from build123d import *
from build123d.topology import SkipClean

# Parameters (mm, degrees)
SKETCH1_W           = 95
SKETCH1_H           = 62
SKETCH1_R           = 1.7
BOSS_EXTRUDE1_DEPTH = 3
SKETCH2_W           = 75
SKETCH2_H           = 52
BOSS_EXTRUDE2_DEPTH = 28.85
SKETCH3_W           = 69
SKETCH3_H           = 25.85
CUT_EXTRUDE1_DEPTH  = 118.827935991
SKETCH4_W           = 69
SKETCH4_H           = 3
CUT_EXTRUDE2_DEPTH  = 118.827935991
SKETCH5_R           = 1.3
SKETCH5_W           = 32
SKETCH5_H           = 14
CUT_EXTRUDE3_DEPTH  = 118.827935991
SKETCH7_R           = 3
CUT_EXTRUDE5_DEPTH  = 118.827935991
SKETCH6_W           = 15
SKETCH6_H           = 9
SKETCH6_W_2         = 8
SKETCH6_H_2         = 10.5
CUT_EXTRUDE4_DEPTH  = 118.827935991
FILLET1_R           = 2
SKETCH8_R           = 2.5
SKETCH8_R_2         = 1.3
BOSS_EXTRUDE4_DEPTH = 4
FILLET2_R           = 5


with BuildPart() as part:
    # Sketch1 → Boss-Extrude1 (new body)
    with BuildSketch(Plane(origin=(0, 0, 0), x_dir=(1, 0, 0), z_dir=(0, 1, 0))):
        with Locations((47.5, 31)):
            Rectangle(SKETCH1_W, SKETCH1_H)
        with Locations(Location((90.04349796, 55.565, 0), (0, 0, 270))):
            Circle(SKETCH1_R, mode=Mode.SUBTRACT)
        with Locations(Location((90.04349796, 6.435, 0), (0, 0, 270))):
            Circle(SKETCH1_R, mode=Mode.SUBTRACT)
        with Locations(Location((4.95650204, 55.565, 0), (0, 0, 270))):
            Circle(SKETCH1_R, mode=Mode.SUBTRACT)
        with Locations(Location((4.95650204, 6.435, 0), (0, 0, 270))):
            Circle(SKETCH1_R, mode=Mode.SUBTRACT)
    extrude(amount=BOSS_EXTRUDE1_DEPTH)

    # Sketch2 → Boss-Extrude2 (add)
    with BuildSketch(Plane(origin=(0, 3, 0), x_dir=(1, 0, 0), z_dir=(0, 1, 0))):
        with Locations((47.5, 26)):
            Rectangle(SKETCH2_W, SKETCH2_H)
    extrude(amount=BOSS_EXTRUDE2_DEPTH)

    # Sketch3 → Cut-Extrude1 (cut, through all)
    with BuildSketch(Plane.XY):
        with Locations((47.5, 15.925)):
            Rectangle(SKETCH3_W, SKETCH3_H)
    extrude(amount=-CUT_EXTRUDE1_DEPTH, mode=Mode.SUBTRACT)

    # Sketch4 → Cut-Extrude2 (cut, through all)
    with BuildSketch(Plane.XY):
        with Locations((47.5, 1.5)):
            Rectangle(SKETCH4_W, SKETCH4_H)
    extrude(amount=-CUT_EXTRUDE2_DEPTH, mode=Mode.SUBTRACT)

    # Sketch5 → Cut-Extrude3 (cut, through all)
    with BuildSketch(Plane(origin=(0, 31.85, 0), x_dir=(1, 0, 0), z_dir=(0, 1, 0))):
        with Locations(Location((27.5, 46, 0), (0, 0, 270))):
            Circle(SKETCH5_R)
        with Locations(Location((27.5, 8, 0), (0, 0, 270))):
            Circle(SKETCH5_R)
        with Locations(Location((67.5, 8, 0), (0, 0, 270))):
            Circle(SKETCH5_R)
        with Locations(Location((67.5, 46, 0), (0, 0, 270))):
            Circle(SKETCH5_R)
        with Locations((47.5, 7)):
            Rectangle(SKETCH5_W, SKETCH5_H)
    extrude(amount=-CUT_EXTRUDE3_DEPTH, mode=Mode.SUBTRACT)

    # Sketch7 → Cut-Extrude5 (cut, through all)
    with BuildSketch(Plane(origin=(0, 31.85, 0), x_dir=(1, 0, 0), z_dir=(0, 1, 0))):
        with Locations((34, 10.8)):
            Circle(SKETCH7_R)
        with Locations((61, 10.8)):
            Circle(SKETCH7_R)
    extrude(amount=-CUT_EXTRUDE5_DEPTH, mode=Mode.SUBTRACT)

    # Sketch6 → Cut-Extrude4 (cut, through all)
    with BuildSketch(Plane(origin=(0, 31.85, 0), x_dir=(1, 0, 0), z_dir=(0, 1, 0))):
        with Locations((38.8, 47.5)):
            Rectangle(SKETCH6_W, SKETCH6_H)
        with Locations((68, 37.75)):
            Rectangle(SKETCH6_W_2, SKETCH6_H_2)
    extrude(amount=-CUT_EXTRUDE4_DEPTH, mode=Mode.SUBTRACT)

    # Fillet1
    fillet1_edges = [part.edges().sort_by_distance(p)[0] for p in [
        (10, 3, -26),
        (85, 3, -26),
        (10, 31.85, -26),
        (85, 31.85, -26),
        (13, 28.85, -26),
        (82, 28.85, -26),
        (13, 0, -31),
        (82, 0, -31),
    ]]
    fillet(fillet1_edges, radius=FILLET1_R)

    # Sketch8 → Boss-Extrude4 (add)
    # profile 1 of 4: a face of its own
    with SkipClean():  # the faces are left unmerged after this step: merging them gives an invalid solid
        with BuildSketch(Plane.XZ.offset(-28.85)):
            with Locations(Location((27.5, -8, 0), (0, 0, 90))):
                Circle(SKETCH8_R)
            with Locations(Location((27.5, -8, 0), (0, 0, 90))):
                Circle(SKETCH8_R_2, mode=Mode.SUBTRACT)
        # profile 2 of 4: a face of its own
        with BuildSketch(Plane.XZ.offset(-28.85)):
            with Locations(Location((67.5, -8, 0), (0, 0, 90))):
                Circle(SKETCH8_R)
            with Locations(Location((67.5, -8, 0), (0, 0, 270))):
                Circle(SKETCH8_R_2, mode=Mode.SUBTRACT)
        # profile 3 of 4: a face of its own
        with BuildSketch(Plane.XZ.offset(-28.85)):
            with Locations(Location((27.5, -46, 0), (0, 0, 90))):
                Circle(SKETCH8_R)
            with Locations(Location((27.5, -46, 0), (0, 0, 90))):
                Circle(SKETCH8_R_2, mode=Mode.SUBTRACT)
        # profile 4 of 4: a face of its own
        with BuildSketch(Plane.XZ.offset(-28.85)):
            with Locations(Location((67.5, -46, 0), (0, 0, 90))):
                Circle(SKETCH8_R)
            with Locations(Location((67.5, -46, 0), (0, 0, 270))):
                Circle(SKETCH8_R_2, mode=Mode.SUBTRACT)
        extrude(amount=BOSS_EXTRUDE4_DEPTH)

    # Fillet2
    fillet2_edges = [part.edges().sort_by_distance(p)[0] for p in [
        (0, 1.5, -62),
        (95, 1.5, -62),
        (95, 1.5, 0),
        (0, 1.5, 0),
    ]]
    fillet(fillet2_edges, radius=FILLET2_R)


solid = part.part
Geometry check sheet. Reference: the model listing, model coordinates, mm. A direction names the side the tool comes from. Round coordinates to 2 decimals unless told otherwise and drop trailing zeros. Order: outer loops, then holes, each group sorted by start corner. A loop starts at its lowest first (then second) coordinate and runs counter-clockwise, first axis right, second up. Notation, with made-up numbers: M -9.5,75 L 26.5,75 A18 cw 26.5,93 Z; hole C 72,48 d1. An arc over 180 degrees is marked long. Write each question's results on one line, items separated by ' | '. Start each with the question number.
1. Cross-section at A-A on x = 67.5. Record the boundary of the cut face in (y, z).
2. Cross-section at C-C on x = 27.5. Record the boundary of the cut face in (y, z), plus the area to 3 significant figures.
3. Set-up check for faces 4 (the face through (81.4, 28.28, -26.36)), 5 (the face through (25, 27, -8)), 6 (the face through (68, 30, -43)), 7 (the face through (46.3, 30, -47)), 8 (the face through (31.5, 30, -5)): record each of +Z, -Z, +X, -X, +Y, -Y from which the full face is reachable in a straight line by a thin tool's end or side.
4. Cross-section at D-D on z = -18. Record the boundary of the cut face in (x, y).
5. Material ranges on L1, parallel to X at y = 26.6, z = -46; L2, parallel to X at y = 23, z = -5; L3, parallel to X at y = 27.6, z = -46, recorded low to high. Write a range as from..to.
6. Go/stop test with flat-tipped pins: P1, Ø12, axis at x = 21.5, y = 25, coming from the -Z side; P2, Ø10.5, axis at x = 4, z = -21, coming from the +Y side; P3, Ø2.5, axis at x = 55, y = 31, coming from the +Z side; P4, Ø2, axis at x = 67.5, z = -46, coming from the -Y side. Record where each tip stops, or that it passes through.
7. Draft check along X on faces 1 (the face through (5.467, 1.479, -53.944)), 2 (the face through (84.4, 31.28, -26.36)), 3 (the face through (1, 2, -60)). Enter one of: pulls with the +X half, pulls with the -X half, needs draft (parallel to the pull), parting line crosses it, or undercut.
8. Cross-section at B-B on y = 21. Record the boundary of the cut face in (x, z), plus the area to 3 significant figures.
Resolved:
1) outline: M 24.85,-48.5 L 28.85,-48.5 L 28.85,-52 L 31.85,-52 L 31.85,-47.3 L 24.85,-47.3 Z; M 24.85,-44.7 L 31.85,-44.7 L 31.85,-43 L 28.85,-43 L 28.85,-43.5 L 24.85,-43.5 Z; M 24.85,-10.5 L 28.85,-10.5 L 28.85,-32.5 L 31.85,-32.5 L 31.85,-9.3 L 24.85,-9.3 Z; M 24.85,-6.7 L 31.85,-6.7 L 31.85,0 L 28.85,0 L 28.85,-5.5 L 24.85,-5.5 Z
2) outline: M 24.85,-48.5 L 28.85,-48.5 L 28.85,-52 L 31.85,-52 L 31.85,-47.3 L 24.85,-47.3 Z; M 24.85,-44.7 L 31.85,-44.7 L 31.85,-9.3 L 24.85,-9.3 L 24.85,-10.5 L 28.85,-10.5 L 28.85,-43.5 L 24.85,-43.5 Z; M 24.85,-6.7 L 31.85,-6.7 L 31.85,0 L 28.85,0 L 28.85,-5.5 L 24.85,-5.5 Z | area: 160 mm2
3) face 4: +Z, -Z, -Y | face 5: -Y | face 6: +Y, -Y | face 7: -Z, +Y, -Y | face 8: +Z, +Y, -Y
4) outline: M 0,0 L 11,0 A2 ccw 13,2 L 13,26.85 A2 cw 15,28.85 L 80,28.85 A2 cw 82,26.85 L 82,2 A2 ccw 84,0 L 95,0 L 95,3 L 87,3 A2 cw 85,5 L 85,29.85 A2 ccw 83,31.85 L 12,31.85 A2 ccw 10,29.85 L 10,5 A2 cw 8,3 L 0,3 Z
5) L1: 10..13, 25..26.2, 28.8..30, 65..66.2, 68.8..70, 82..85 | L2: 10..13, 82..85 | L3: 10..13.15, 25..26.2, 28.8..30, 65..66.2, 68.8..70, 81.85..85
6) P1: z = -52 | P2: y = 3.44 | P3: z = -14 | P4: through
7) face 1: undercut | face 2: pulls with the +X half | face 3: pulls with the -X half
8) outline: M 10,-52 L 13,-52 L 13,0 L 10,0 Z; M 82,-52 L 85,-52 L 85,0 L 82,0 Z | area: 312 mm2
